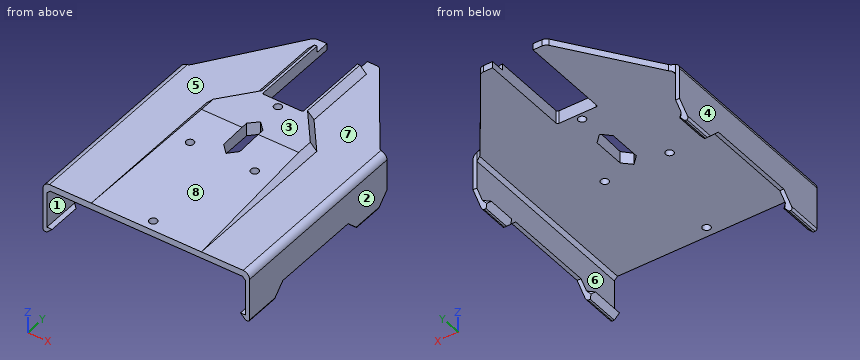
```python
from build123d import *

# Parameters (mm, degrees)
PAD002_DEPTH         = 119
PAD003_DEPTH         = 17
POCKET015_DEPTH      = 119.001
SKETCH040_R          = 1.2
POCKET016_DEPTH      = 20.8744738654
POCKET017_DEPTH      = 16.001
POCKET018_DEPTH      = 16.001
POCKET018_DEPTH_BACK = 1.601
SKETCH044_R          = 1.2
POCKET019_DEPTH      = 1.601
POCKET019_DEPTH_BACK = 16.001
POCKET020_DEPTH      = 27.001
SKETCH048_W          = 4.3
SKETCH048_H          = 2
POCKET021_DEPTH      = 31.9010001
POCKET021_DEPTH_BACK = 31.9010001
POCKET023_DEPTH      = 31.9010001
POCKET023_DEPTH_BACK = 31.9010001
POCKET024_DEPTH      = 1.601


with BuildPart() as part:
    # Sketch033 → Pad002 (new body)
    with BuildSketch(Plane.XZ):
        with BuildLine():
            Line((-30.7, 11), (-30.7, 0))
            Line((-30.7, 0), (-29.1, 0))
            Line((-29.1, 0), (-30.7, -1.6))
            Line((-30.7, -1.6), (-31.3, -1.6))
            ThreePointArc((-31.9, -1), (-31.7242640687, -1.4242640687), (-31.3, -1.6))
            Line((-31.9, -1), (-31.9, 12))
            ThreePointArc((-29.9, 14), (-31.3142135624, 13.4142135624), (-31.9, 12))
            Line((-29.9, 14), (29.9, 14))
            ThreePointArc((31.9, 12), (31.3142135624, 13.4142135624), (29.9, 14))
            Line((31.9, -1), (31.9, 12))
            ThreePointArc((31.3, -1.6), (31.7242640687, -1.4242640687), (31.9, -1))
            Line((30.7, -1.6), (31.3, -1.6))
            Line((29.1, 0), (30.7, -1.6))
            Line((30.7, 0), (29.1, 0))
            Line((30.7, 11), (30.7, 0))
            Line((29.7, 12), (30.7, 11))
            Line((-29.7, 12), (29.7, 12))
            Line((-30.7, 11), (-29.7, 12))
        make_face()
    extrude(amount=-PAD002_DEPTH)

    # Sketch034 → Pad003 (join, symmetric)
    with BuildSketch(Plane.YZ):
        Polygon((0, 14), (119, 14), (119, 16), (44.955533586, 16), align=None)
    extrude(amount=PAD003_DEPTH, both=True)

    # Sketch039 → Pocket015 (cut, through all)
    with BuildSketch(Plane.XZ):
        Polygon((-17, 14), (-15, 16), (15, 16), (17, 14), (31.9, 14), (31.9, 26), (-31.9, 26), (-31.9, 14), align=None)
    extrude(amount=-POCKET015_DEPTH, mode=Mode.SUBTRACT)

    # Sketch040 (on DatumPlane) → Pocket016 (cut, through all)
    with BuildSketch(Plane(origin=(0, 0, 14), x_dir=(1, 0, 0), z_dir=(0, -0.0444444444, 0.9990118575))):
        with Locations((-10, 33)):
            Circle(SKETCH040_R)
        with Locations((10, 33)):
            Circle(SKETCH040_R)
        with Locations((0, 3)):
            Circle(SKETCH040_R)
    extrude(amount=-POCKET016_DEPTH, mode=Mode.SUBTRACT)

    # Sketch041 → Pocket017 (cut, through all)
    with BuildSketch(Plane.XY):
        Polygon((0, 49.5), (-2.5, 47), (-2.5, 37), (0, 34.5), (2.5, 37), (2.5, 47), align=None)
    extrude(amount=POCKET017_DEPTH, mode=Mode.SUBTRACT)

    # Sketch043 → Pocket018 (cut, two sides)
    with BuildSketch(Plane.XY) as pocket018_sk:
        with BuildLine():
            Line((-9, 87), (9, 87))
            ThreePointArc((10.6275065469, 86.1624209391), (9.9151934555, 86.7783196954), (9, 87))
            Line((10.6275065469, 86.1624209391), (29.0724934531, 60.3375790609))
            ThreePointArc((29.0724934531, 60.3375790609), (29.7848065445, 59.7216803046), (30.7, 59.5))
            Line((30.7, 59.5), (61.4, 59.5))
            Line((61.4, 119), (61.4, 59.5))
            Line((-61.4, 119), (61.4, 119))
            Line((-61.4, 59.5), (-61.4, 119))
            Line((-30.7, 59.5), (-61.4, 59.5))
            ThreePointArc((-30.7, 59.5), (-29.7848065445, 59.7216803046), (-29.0724934531, 60.3375790609))
            Line((-10.6275065469, 86.1624209391), (-29.0724934531, 60.3375790609))
            ThreePointArc((-9, 87), (-9.9151934555, 86.7783196954), (-10.6275065469, 86.1624209391))
        make_face()
    extrude(amount=POCKET018_DEPTH, mode=Mode.SUBTRACT)
    extrude(pocket018_sk.sketch, amount=-POCKET018_DEPTH_BACK, mode=Mode.SUBTRACT)

    # Sketch044 → Pocket019 (cut, two sides)
    with BuildSketch(Plane.XY) as pocket019_sk:
        with Locations((0, 57)):
            Circle(SKETCH044_R)
        with BuildLine():
            Line((-6.25, 119), (6.25, 119))
            Line((6.25, 119), (6.25, 59.5))
            ThreePointArc((5.75, 59), (6.1035533906, 59.1464466094), (6.25, 59.5))
            Line((5.75, 59), (-5.75, 59))
            ThreePointArc((-6.25, 59.5), (-6.1035533906, 59.1464466094), (-5.75, 59))
            Line((-6.25, 59.5), (-6.25, 119))
        make_face()
    extrude(amount=-POCKET019_DEPTH, mode=Mode.SUBTRACT)
    extrude(pocket019_sk.sketch, amount=POCKET019_DEPTH_BACK, mode=Mode.SUBTRACT)

    # Sketch045 (on DatumPlane) → SubtractiveLoft001 section 0
    with BuildSketch(Plane.XZ.offset(-50)):
        Polygon((-17, 14), (-15, 16), (15, 16), (17, 14), (31.9, 14), (31.9, 26), (-31.9, 26), (-31.9, 14), align=None)
    # Sketch046 (on DatumPlane) → SubtractiveLoft001 section 1
    with BuildSketch(Plane.XZ.offset(-60)):
        Polygon((-9, 14), (-7, 16), (7, 16), (9, 14), (31.9, 14), (31.9, 26), (-31.9, 26), (-31.9, 14), align=None)
    loft(mode=Mode.SUBTRACT)

    # Sketch047 (on DatumPlane) → Pocket020 (cut, through all)
    with BuildSketch(Plane.XZ.offset(-60)):
        Polygon((-9, 14), (-7, 16), (7, 16), (9, 14), (31.9, 14), (31.9, 26), (-31.9, 26), (-31.9, 14), align=None)
    extrude(amount=-POCKET020_DEPTH, mode=Mode.SUBTRACT)

    # Sketch048 → Pocket021 (cut, two sides)
    with BuildSketch(Plane.YZ) as pocket021_sk:
        with Locations((84.85, 15)):
            Rectangle(SKETCH048_W, SKETCH048_H)
    extrude(amount=-POCKET021_DEPTH, mode=Mode.SUBTRACT)
    extrude(pocket021_sk.sketch, amount=POCKET021_DEPTH_BACK, mode=Mode.SUBTRACT)

    # Sketch051 → Pocket023 (cut, two sides)
    with BuildSketch(Plane.YZ) as pocket023_sk:
        Polygon((0, -1.6), (10.4, -1.6), (14.4, 2.4), (42.7, 2.4), (46.7, -1.6), (55.5, -1.6), (59.5, 2.4), (63.5, 2.4), (63.5, -13.6), (0, -13.6), align=None)
    extrude(amount=-POCKET023_DEPTH, mode=Mode.SUBTRACT)
    extrude(pocket023_sk.sketch, amount=POCKET023_DEPTH_BACK, mode=Mode.SUBTRACT)

    # Sketch052 → Pocket024 (cut, through all)
    with BuildSketch(Plane.XY):
        Polygon((-29.1, 10.4), (29.1, 10.4), (30.7, 12), (30.7, 45.1), (29.1, 46.7), (29.1, 55.5), (30.7, 57.1), (30.7, 69.1), (-30.7, 69.1), (-30.7, 57.1), (-29.1, 55.5), (-29.1, 46.7), (-30.7, 45.1), (-30.7, 12), align=None)
    extrude(amount=-POCKET024_DEPTH, mode=Mode.SUBTRACT)


with BuildPart() as part_1:
    # Body002 placement: moved
    add(part.part.moved(Location((0, 18, 5))))


solid = part_1.part
```
Model file for the job. Use its own axes, mm. Face numbers are marked on the shaded views. A direction names the side the tool comes from. Coordinates: 2 decimals unless noted, no trailing zeros. Loops run counter-clockwise (first coordinate to the right, second up) from the corner with the lowest first, then second, coordinate; pieces in that order, holes last. Notation, with made-up numbers: (74, -18) -> (113, -18) arc R29 ccw to (113, 2) -> close; hole circle Ø9 at (33, -37.5). An arc over 180 degrees is marked (long way). Answer as a JSON object with one key per item and string values.
Q1. Flat gauge pins, fed straight in: P1, Ø1.8, axis at x = 30, y = 23.5, coming from the +Z side; P2, Ø0.6, axis at x = 31.5, z = 16, coming from the +Y side; P3, Ø8, axis at x = -21, z = 19, coming from the +Y side. Where does each tip first touch, or does it go through?
Report:
{"P1": "stops at z = 19", "P2": "stops at y = 77.5", "P3": "stops at y = 95.24"}
Q2. Cut at D-D (y = 26). List the corners of the cut face in (x, z).
Report:
{"outline": "(-31.9, 4) arc R0.6 ccw to (-31.3, 3.4) -> (-30.7, 3.4) -> (-29.1, 5) -> (-30.7, 5) -> (-30.7, 16) -> (-29.7, 17) -> (29.7, 17) -> (30.7, 16) -> (30.7, 5) -> (29.1, 5) -> (30.7, 3.4) -> (31.3, 3.4) arc R0.6 ccw to (31.9, 4) -> (31.9, 17) arc R2 ccw to (29.9, 19) -> (17, 19) -> (16.64, 19.36) -> (-16.64, 19.36) -> (-17, 19) -> (-29.9, 19) arc R2 ccw to (-31.9, 17) -> close"}
Q3. Pull direction X, two halves, no side cores. Call the marked faces 1, 2 and 3: released by +X, released by -X, zero draft, split by the parting line, or undercut.
Report:
{"face 1": "undercut", "face 2": "released by +X", "face 3": "zero draft"}
Q4. Cut at A-A (z = 14). List the corners of the cut face in (x, y).
Report:
{"outline": "(-31.9, 18) -> (-30.7, 18) -> (-30.7, 77.5) -> (-31.9, 77.5) -> close; (30.7, 18) -> (31.9, 18) -> (31.9, 77.5) -> (30.7, 77.5) -> close"}
Q5. Probe probe 1 along X at (y, z) = (60, 15.25); probe 2 along Z at (x, y) = (24.5, 35); probe 3 along X at (y, z) = (75, 19.4). List the from-to ranges inside material, lowest first.
Report:
{"probe 1": "x = -31.9 to -30.7, 30.7 to 31.9", "probe 2": "z = 17 to 19", "probe 3": "x = -11 to -1.2, 1.2 to 11"}
Q6. Cut at C-C (y = 56.5). List the corners of the cut face in (x, z), and give its area (3 significant figures).
Report:
{"outline": "(-31.9, 7.4) -> (-30.7, 7.4) -> (-30.7, 16) -> (-29.7, 17) -> (-2.5, 17) -> (-2.5, 20.71) -> (-15.29, 20.71) -> (-17, 19) -> (-29.9, 19) arc R2 ccw to (-31.9, 17) -> close; (2.5, 17) -> (29.7, 17) -> (30.7, 16) -> (30.7, 7.4) -> (31.9, 7.4) -> (31.9, 17) arc R2 ccw to (29.9, 19) -> (17, 19) -> (15.29, 20.71) -> (2.5, 20.71) -> close", "area": "187 mm2"}
Q7. Cut at B-B (z = 6). List the corners of the cut face in (x, y).
Report:
{"outline": "(-31.9, 18) -> (-30.7, 18) -> (-30.7, 31) -> (-31.9, 31) -> close; (-31.9, 62.1) -> (-30.7, 62.1) -> (-30.7, 76.1) -> (-31.9, 76.1) -> close; (30.7, 18) -> (31.9, 18) -> (31.9, 31) -> (30.7, 31) -> close; (30.7, 62.1) -> (31.9, 62.1) -> (31.9, 76.1) -> (30.7, 76.1) -> close"}
Q8. 3-axis set-ups, long thin cutter, end or side, ignore diameter. For the marked faces 4, 5, 6, 7 and 8: which of +Z, -Z, +X, -X, +Y, -Y reach the whole face in a straight line?
Report:
{"face 4": "+Z, -Z, -X, +Y, -Y", "face 5": "+Z, -X, +Y", "face 6": "+Y, -Y", "face 7": "+Z, +X, +Y", "face 8": "+Z, +X, -X, -Y"}
